```python
from build123d import *


with BuildPart() as part:
    # Esquisse1 → Base-Révolution (revolve)
    with BuildSketch(Plane.XY, mode=Mode.PRIVATE) as base_r_volution_sk:
        with BuildLine():
            Line((0, 13.1), (0, 18.25))
            Line((0, 18.25), (-3.385649604, 17.342817923))
            Line((-3.385649604, 17.342817923), (-3.108014609, 16.306670018))
            Line((-3.108014609, 16.306670018), (-12.11177275, 14.186566402))
            Line((-12.11177275, 14.186566402), (-12.316296218, 14.949858375))
            Line((-12.316296218, 14.949858375), (-15, 14.230762114))
            Line((-15, 14.230762114), (-15, 13.1))
            ThreePointArc((-15, 13.1), (-14.824264069, 12.675735931), (-14.4, 12.5))
            Line((-14.4, 12.5), (-0.6, 12.5))
            ThreePointArc((-0.6, 12.5), (-0.175735931, 12.675735931), (0, 13.1))
        make_face()
    revolve(base_r_volution_sk.sketch.rotate(Axis((0, 0, 0), (-1, 0, 0)), 90), axis=Axis((0, 0, 0), (-1, 0, 0)))


solid = part.part
```
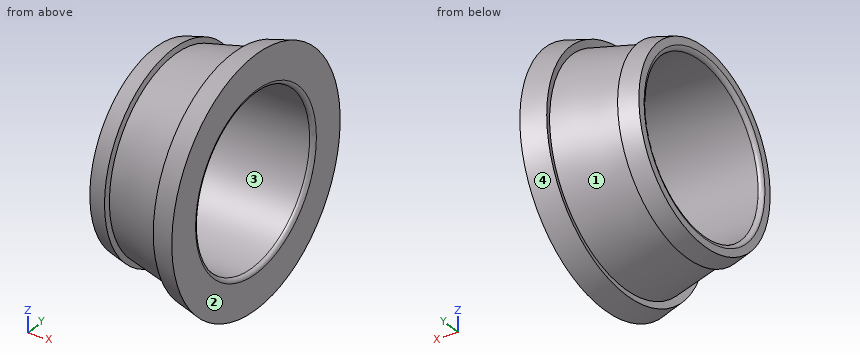
Work out the finished part from the listing and answer in its coordinate system (mm). Face numbers are marked on the shaded views. Round coordinates to 2 decimals unless told otherwise and drop trailing zeros. Loops run counter-clockwise (first coordinate to the right, second up) from the corner with the lowest first, then second, coordinate; pieces in that order, holes last. Notation, with made-up numbers: M -28,-15 L 29,-15 A18 cw 29,9 Z; hole C 61.5,70 d11. An arc over 180 degrees is marked long. One line per question, with ' | ' between items.
Q1. Consider line 1 along Y through (x, z) = (-4, 3); line 2 along Y through (x, z) = (-4.5, 4.5); line 3 along Z through (x, y) = (-2.75, 5). Determine where each line is inside the solid, lowest interval first. Write a range as from..to.
Conclusion:
line 1: y = -15.81..-12.13, 12.13..15.81 | line 2: y = -15.33..-11.66, 11.66..15.33 | line 3: z = -16.78..-11.46, 11.46..16.78
Q2. Find section D-D, the plane x = -6.25. Give the vertices of the cut face in (y, z), then the cut area to 3 significant figures.
Conclusion:
outline: C 0,0 d31.13; hole C 0,0 d25 | area: 270 mm2
Q3. Find section C-C, the plane x = -9.5. Give the vertices of the cut face in (y, z).
Conclusion:
outline: C 0,0 d29.6; hole C 0,0 d25
Q4. The mould has two halves that part along X. Classify the marked faces 1, 2, 3 and 4: +X half, -X half, draft (parallel to the pull), parting line (faces both ways), or undercut.
Conclusion:
face 1: undercut | face 2: +X half | face 3: draft | face 4: -X half
Q5. Each of these flat-tipped pins is pushed along its axis until it touches: pin 1 Ø1 at (x, y) = (-2.5, -13.5) entering from +Z; pin 2 Ø2 at (x, y) = (-11, -10.5) entering from +Z; pin 3 Ø1.5 at (x, y) = (-12, 1.5) entering from -Z. Where does it stop, or does it pass through?
Conclusion:
pin 1: stops at z = 11.87 | pin 2: stops at z = 10.94 | pin 3: stops at z = -14.93
Q6. Find section A-A, the plane y = 0. Give the vertices of the cut face in (x, z).
Conclusion:
outline: M -15,-14.23 L -12.32,-14.95 L -12.11,-14.19 L -3.11,-16.31 L -3.39,-17.34 L 0,-18.25 L 0,-13.1 A0.6 ccw -0.6,-12.5 L -14.4,-12.5 A0.6 ccw -15,-13.1 Z; M -15,13.1 A0.6 ccw -14.4,12.5 L -0.6,12.5 A0.6 ccw 0,13.1 L 0,18.25 L -3.39,17.34 L -3.11,16.31 L -12.11,14.19 L -12.32,14.95 L -15,14.23 Z
